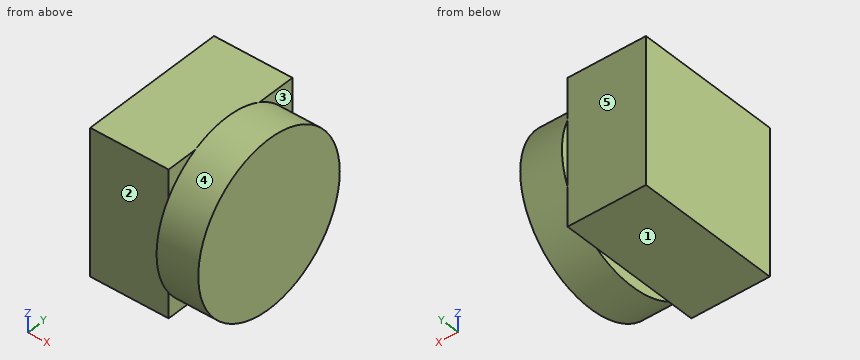
```python
from build123d import *

# Parameters (mm, degrees)
F0_W     = 22.225
F0_H     = 22.225
F0_R     = 5.08
F1_DEPTH = 11.938
F2_DEPTH = 18.288
F4_R     = 12.7
F5_DEPTH = 6.35


with BuildPart() as f1:
    # F0 (on Right) → F1 (new body)
    with BuildSketch(Plane.YZ):
        with Locations((-4.1858740151, 25.9753634954)):
            Rectangle(F0_W, F0_H)
        with Locations((-4.1858740151, 25.9753634954)):
            Circle(F0_R, mode=Mode.SUBTRACT)
    extrude(amount=F1_DEPTH)

    # F0 (on Right) → F2 (join)
    with BuildSketch(Plane.YZ):
        with Locations((-4.1858740151, 25.9753634954)):
            Circle(F0_R)
    extrude(amount=F2_DEPTH)

    # F4 (on offset) → F5 (join)
    with BuildSketch(Plane.YZ.offset(11.938)):
        with Locations((-4.7678221017, 25.7760342211)):
            Circle(F4_R)
    extrude(amount=F5_DEPTH)


solid = f1.part
```
Verification items for the finished model (mm, model axes). Face numbers are marked on the shaded views. A direction names the side the tool comes from. Coordinates: 2 decimals unless noted, no trailing zeros. Loops run counter-clockwise (first coordinate to the right, second up) from the corner with the lowest first, then second, coordinate; pieces in that order, holes last. Notation, with made-up numbers: (-37.5, -22) -> (-18.5, -22) arc R8 ccw to (-18.5, -10) -> close; hole circle Ø8 at (43.25, 86). An arc over 180 degrees is marked (long way). Answer in a Markdown table with one row per item. Add a question column.
1. Section check D-D, the plane y = -16. Enter the section's corners in (x, z), then the cut area to 3 significant figures.
2. Depth check by flat-ended pin: P1, Ø1, axis at x = 8.5, y = 3, coming from the +Z side; P2, Ø8, axis at x = 6.5, z = 28.5, coming from the -Y side; P3, Ø3.5, axis at x = 3.5, z = 25, coming from the +Y side. Enter the tip coordinate at first touch or a pass-through.
3. Material ranges on probe 1 along Z at (x, y) = (1.5, -1.75); probe 2 along Y at (x, z) = (6, 30); probe 3 along X at (y, z) = (-15.75, 22.5), recorded low to high. Write a range as [from, to].
4. Section check B-B, the plane y = 3.25. Enter the section's corners in (x, z).
5. Access from +Z, -Z, +X, -X, +Y, -Y to the whole of each face (thin tool, end or side, straight path). Record for the marked faces 1, 2, 3, 4 and 5.
6. Section check A-A, the plane z = 19.5. Enter the section's corners in (x, y), then the cut area to 3 significant figures.
7. Section check C-C, the plane x = 4.5. Enter the section's corners in (y, z).
Derived:
| question | item | result |
|---|---|---|
| 1 | outline | (11.94, 19.85) -> (18.29, 19.85) -> (18.29, 31.7) -> (11.94, 31.7) -> close |
| 1 | area | 75.3 mm² |
| 2 | P1 | stops at z = 37.09 |
| 2 | P2 | stops at y = -15.3 |
| 2 | P3 | stops at y = 6.93 |
| 3 | probe 1 | z = [14.86, 37.09] |
| 3 | probe 2 | y = [-15.3, 6.93] |
| 3 | probe 3 | x = [11.94, 18.29] |
| 4 | outline | (0, 14.86) -> (11.94, 14.86) -> (11.94, 15.93) -> (18.29, 15.93) -> (18.29, 35.63) -> (11.94, 35.63) -> (11.94, 37.09) -> (0, 37.09) -> close |
| 5 | face 1 | -Z, -X, +Y, -Y |
| 5 | face 2 | +Z, -Z, -X, -Y |
| 5 | face 3 | +Z, +X, +Y |
| 5 | face 4 | +X |
| 5 | face 5 | +Z, -Z, -X, +Y |
| 6 | outline | (0, -15.3) -> (11.94, -15.3) -> (11.94, -15.81) -> (18.29, -15.81) -> (18.29, 6.27) -> (11.94, 6.27) -> (11.94, 6.93) -> (0, 6.93) -> close |
| 6 | area | 406 mm² |
| 7 | outline | (-15.3, 14.86) -> (6.93, 14.86) -> (6.93, 37.09) -> (-15.3, 37.09) -> close |
